Can you work these out from the model? Positions are in its coordinate system, mm. A direction names the side the tool comes from. Give positions to 0.01 mm unless a question says otherwise; leave off trailing zeros. Write each loop counter-clockwise with the first axis right and the second up, starting at its lowest first coordinate (ties: lowest second). Pieces come first, ordered by that corner, then holes.
Autodesk Inventor part; units mm, degrees
ref_plane "YZ Plane" through (0, 0, 0) normal (1, 0, 0) x (0, 1, 0)
ref_plane "XZ Plane" through (0, 0, 0) normal (0, 1, 0) x (-1, 0, 0)
ref_plane "XY Plane" through (0, 0, 0) normal (0, 0, 1) x (1, 0, 0)
sketch "Sketch1" plane through (0, 0, 0) normal (0, 0, 1) x (1, 0, 0)
  circle A0 centre (0, 0) radius 18.4
  circle A1 centre (0, 0) radius 13
  circle A2 centre (0, -7) radius 6
  circle A3 centre (0, -7) radius 3
  circle A4 centre (0, 0) radius 15.5
  circle A5 centre (0, 15.5) radius 1.6
  circle A6 centre (7.75, 13.4234) radius 1.6
  circle A7 centre (-7.75, 13.4234) radius 1.6
  circle A8 centre (-15.5, 0) radius 1.6
  circle A9 centre (-13.4234, -7.75) radius 1.6
  circle A10 centre (-7.75, -13.4234) radius 1.6
  circle A11 centre (15.5, 0) radius 1.6
  circle A12 centre (13.4234, -7.75) radius 1.6
  circle A13 centre (7.75, -13.4234) radius 1.6
  dimension "d0" = 36.8
  dimension "d1" = 6
  dimension "d3" = 12
  dimension "d16" = 3.2
  dimension "d17" = 15.5
  dimension "d19" = 8.0234
  dimension "d20" = 8.0234
  dimension "d21" = 8.0234
  dimension "d22" = 8.0234
  dimension "d25" = 31
  dimension "d26" = 31
  dimension "d27" = 31
  dimension "d28" = 15.5
  dimension "d29" = 15.5
  dimension "d30" = 8.0234
  dimension "d31" = 8.0234
  dimension "d32" = 7
extrude "Extrusion1" add sketch "Sketch1" against normal blind 64.516 contours A0 | A2 | A1 | A3 | A4 A11 | A4 A11 | A11 A4 A12 A13 A10 A9 A8 A7 A5 A6 | A6 A4 | A4 A6 | A12 A4 | A4 A12 | A5 A4 | A4 A5 | A13 A4 | A4 A13 | A7 A4 | A4 A7 | A10 A4 | A4 A10 | A8 A4 | A4 A8 | A9 A4 | A4 A9
extrude "Extrusion2" add sketch "Sketch1" along normal blind 6.5 contours A2
extrude "Extrusion3" add sketch "Sketch1" along normal blind 15.5 contours A3
sketch "Sketch2" plane through (0, 0, -64.516) normal (0, 0, -1) x (-1, 0, 0)
  circle A0 centre (0, 0) radius 18.4
  circle A1 centre (0, 0) radius 12.05
  dimension "d10" = 24.1
extrude "Extrusion4" add sketch "Sketch2" along normal blind 5.6 contours A1
chamfer "Chamfer1" distance 1 angle 45 1 edges at (-6, -7, 6.5)
extrude "Extrusion5" cut sketch "Sketch1" against normal blind 1 contours A1
extrude "Extrusion6" cut sketch "Sketch1" against normal blind 10 contours A4 A11 | A4 A11 | A6 A4 | A4 A6 | A12 A4 | A4 A12 | A5 A4 | A4 A5 | A13 A4 | A4 A13 | A7 A4 | A4 A7 | A10 A4 | A4 A10 | A8 A4 | A4 A8 | A9 A4 | A4 A9
equation "\"d19\" = d20"
equation "\"d21\" = d19"
equation "\"d22\" = d21"
equation "\"d26\" = d25"
equation "\"d27\" = d25"
equation "\"d28\" = d17"
equation "\"d30\" = d19"
properties part number "motor"
1) If we mould it in two halves opening along Y, with no side actions, what happens to faces 1 (the face through (-14.6, -11.2, -31.8)), 2 (the face through (0, 3, -1)), 3 (the face through (3.3, -6.9, 6.5))? For each: +Y half, -Y half, draft (parallel to the pull), parting line (faces both ways), or undercut.
Values follow:
face 1: parting line
face 2: undercut
face 3: draft
2) For pin 1 Ø6 at (x, z) = (-13.5, -14) entering from +Y; pin 2 Ø8 at (x, y) = (-8, -11.5) entering from +Z; pin 3 Ø8 at (y, z) = (5.5, -61) entering from +X, each with a flat end and sliding along its axis, tell me the tip position at first contact or that it passes through.
Values follow:
pin 1: stops at y = 15.11
pin 2: stops at z = 6.32
pin 3: stops at x = 18.34
3) For faces 4 (the face through (8.881, -8.144, -67.277)), 5 (the face through (5.4, -12.2, 0)), which set-ups out of +Z, -Z, +X, -X, +Y, -Y let a thin tool reach every point of the face, with its end or its side?
Values follow:
face 4: -Z
face 5: +Z
4) Please list where these lines run through material, in increasing order: L1, parallel to Y at x = -7.75, z = -7; L2, parallel to Z at x = -9, y = -11.5; L3, parallel to X at y = 15.5, z = -6.25.
Values follow:
L1: y = -16.69 to -15.02, -11.82 to 11.82, 15.02 to 16.69
L2: z = -64.52 to 0
L3: x = -9.92 to -1.6, 1.6 to 9.92
5) Suppose I cut it at A-A on x = -7.75. Write out the boundary of the cut face in (y, z), plus the area to 3 significant figures.
Values follow:
outline: (-16.69, -64.52) - (-9.23, -64.52) - (-9.23, -70.12) - (9.23, -70.12) - (9.23, -64.52) - (16.69, -64.52) - (16.69, 0) - (15.02, 0) - (15.02, -10) - (11.82, -10) - (11.82, 0) - (10.44, 0) - (10.44, -1) - (-10.44, -1) - (-10.44, 0) - (-11.82, 0) - (-11.82, -10) - (-15.02, -10) - (-15.02, 0) - (-16.69, 0) - close
area: 2,170 mm2
6) Suppose I cut it at C-C on y = 8. Write out the boundary of the cut face in (x, z).
Values follow:
outline: (-16.57, -64.52) - (-9.01, -64.52) - (-9.01, -70.12) - (9.01, -70.12) - (9.01, -64.52) - (16.57, -64.52) - (16.57, 0) - (10.25, 0) - (10.25, -1) - (-10.25, -1) - (-10.25, 0) - (-16.57, 0) - close
7) Suppose I cut it at B-B on z = -46. Write out the boundary of the cut face in (x, y).
Values follow:
outline: circle Ø36.8 at (0, 0)
